from build123d import *

# Parameters (mm, degrees)
EXTRUDE_1_DEPTH      = 18
EXTRUDE_2_DEPTH      = 11
SKETCH_3_R           = 1
SKETCH_3_R_2         = 1.5
CUT_EXTRUDE_1_DEPTH  = 31
SKETCH_4_R           = 3
CUT_EXTRUDE_2_DEPTH  = 7
CUT_EXTRUDE_START    = -7
SKETCH_5_R           = 3
CUT_EXTRUDE_3_DEPTH  = 7
SKETCH_6_R           = 2.5
EXTRUDE_3_DEPTH      = 16
CUT_EXTRUDE_START_2  = -9
CUT_EXTRUDE_4_DEPTH  = 9
EXTRUDE_START        = 16
SKETCH_8_R           = 2.5
EXTRUDE_4_DEPTH      = 16
CUT_EXTRUDE_5_DEPTH  = 9
EXTRUDE_5_DEPTH      = 5
SKETCH_11_R          = 1
CUT_EXTRUDE_6_DEPTH  = 14
SKETCH_12_R          = 2
EXTRUDE_6_DEPTH      = 2
SKETCH_13_R          = 2
CUT_EXTRUDE_7_DEPTH  = 5
EXTRUDE_START_2      = 3
SKETCH_14_R          = 1.4
EXTRUDE_8_DEPTH      = 3
CUT_EXTRUDE_8_DEPTH  = 22
CUT_EXTRUDE_9_DEPTH  = 11
SKETCH_18_W          = 4.5245364
SKETCH_18_H          = 2
EXTRUDE_9_DEPTH      = 3
SKETCH_19_W          = 2
SKETCH_19_H          = 1
CUT_EXTRUDE_10_DEPTH = 8
SKETCH_20_W          = 2
SKETCH_20_H          = 1
CUT_EXTRUDE_11_DEPTH = 8
EXTRUDE_START_3      = 25
EXTRUDE_10_DEPTH     = 25
CUT_EXTRUDE_13_DEPTH = 1
EXTRUDE_11_DEPTH     = 3
EXTRUDE_11_DRAFT     = 20
SKETCH_25_R          = 5
EXTRUDE_12_DEPTH     = 2
CUT_EXTRUDE_START_3  = -2
CUT_EXTRUDE_14_DEPTH = 2
CUT_EXTRUDE_START_4  = -14
CUT_EXTRUDE_15_DEPTH = 14
CUT_EXTRUDE_16_DEPTH = 14
SKETCH_32_R          = 1
EXTRUDE_13_DEPTH     = 1


with BuildPart() as part:
    # 草图1 → 凸台-拉伸1 (new body)
    with BuildSketch(Plane.XY):
        with BuildLine():
            Line((0, 0), (-8, 0))
            ThreePointArc((-8, 0), (-10.121320344, 0.878679656), (-11, 3))
            Line((-11, 3), (-11, 32))
            Line((-11, 32), (11, 32))
            Line((11, 32), (11, 3))
            ThreePointArc((11, 3), (10.121320344, 0.878679656), (8, 0))
            Line((8, 0), (0, 0))
        make_face()
    extrude(amount=EXTRUDE_1_DEPTH)

    # 草图2 → 凸台-拉伸2 (add)
    with BuildSketch(Plane(origin=(0, 32, 0), x_dir=(1, 0, 0), z_dir=(0, 1, 0))):
        with BuildLine():
            Line((7.5, -18), (-7.5, -18))
            ThreePointArc((-7.5, -18), (-11.02081528, -9.5), (-7.5, -1))
            Line((-7.5, -1), (0, -1))
            Line((0, -1), (7.5, -1))
            ThreePointArc((7.5, -1), (11.02081528, -9.5), (7.5, -18))
        make_face()
    extrude(amount=EXTRUDE_2_DEPTH)

    # 草图3 → 切除-拉伸1 (cut)
    with BuildSketch(Plane.XY.offset(18)):
        with Locations((9, 30)):
            Circle(SKETCH_3_R)
        with Locations((8.5, 26.5)):
            Circle(SKETCH_3_R_2)
        with Locations((-8.5, 26.5)):
            Circle(SKETCH_3_R_2)
        with Locations((-9, 30)):
            Circle(SKETCH_3_R)
    extrude(amount=-CUT_EXTRUDE_1_DEPTH, mode=Mode.SUBTRACT)

    # 草图4 → 切除-拉伸2 (cut)
    with BuildSketch(Plane.XY.offset(18)):
        with Locations((0, 13)):
            Circle(SKETCH_4_R)
    extrude(amount=-CUT_EXTRUDE_2_DEPTH, mode=Mode.SUBTRACT)

    # 草图5 → 切除-拉伸3 (cut)
    with BuildSketch(Plane(origin=(0, 0, 0), x_dir=(-1, 0, 0), z_dir=(0, 0, -1)).offset(CUT_EXTRUDE_START)):
        with Locations(Location((0, 13, 0), (0, 0, 180))):
            Circle(SKETCH_5_R)
    extrude(amount=CUT_EXTRUDE_3_DEPTH, mode=Mode.SUBTRACT)

    # 草图6 → 凸台-拉伸3 (add)
    with BuildSketch(Plane.XY.offset(11)):
        with Locations((0, 13)):
            Circle(SKETCH_6_R)
    extrude(amount=EXTRUDE_3_DEPTH)

    # 草图7 → 切除-拉伸4 (cut)
    with BuildSketch(Plane.XY.offset(27).offset(CUT_EXTRUDE_START_2)):
        with BuildLine():
            Line((0, 15.5), (2.5, 13))
            ThreePointArc((2.5, 13), (1.767766953, 14.767766953), (0, 15.5))
        make_face()
        with BuildLine():
            Line((-2.5, 13), (0, 10.5))
            ThreePointArc((0, 10.5), (-1.767766953, 11.232233047), (-2.5, 13))
        make_face()
    extrude(amount=CUT_EXTRUDE_4_DEPTH, mode=Mode.SUBTRACT)

    # 草图8 → 凸台-拉伸4 (add)
    with BuildSketch(Plane(origin=(0, 0, 7), x_dir=(-1, 0, 0), z_dir=(0, 0, -1)).offset(EXTRUDE_START)):
        with Locations(Location((0, 13, 0), (0, 0, 180))):
            Circle(SKETCH_8_R)
    extrude(amount=-EXTRUDE_4_DEPTH)

    # 草图9 → 切除-拉伸5 (cut)
    with BuildSketch(Plane(origin=(0, 0, -9), x_dir=(-1, 0, 0), z_dir=(0, 0, -1))):
        with BuildLine():
            Line((0, 15.5), (2.5, 13))
            ThreePointArc((2.5, 13), (1.767766953, 14.767766953), (0, 15.5))
        make_face()
        with BuildLine():
            Line((-2.5, 13), (0, 10.5))
            ThreePointArc((0, 10.5), (-1.767766953, 11.232233047), (-2.5, 13))
        make_face()
    extrude(amount=-CUT_EXTRUDE_5_DEPTH, mode=Mode.SUBTRACT)

    # 草图10 → 凸台-拉伸5 (add)
    with BuildSketch(Plane.XZ):
        Polygon((-2.5, 9), (-2.5, 10.5), (2.5, 10.5), (2.5, 7.5), (-2.5, 7.5), align=None)
    extrude(amount=EXTRUDE_5_DEPTH)

    # 草图11 → 切除-拉伸6 (cut)
    with BuildSketch(Plane.XY.offset(10.5)):
        with Locations((0, -2.5)):
            Circle(SKETCH_11_R)
    extrude(amount=-CUT_EXTRUDE_6_DEPTH, mode=Mode.SUBTRACT)

    # 草图12 → 凸台-拉伸6 (add)
    with BuildSketch(Plane(origin=(0, 0, 0), x_dir=(-1, 0, 0), z_dir=(0, 0, -1))):
        with Locations(Location((0, 22, 0), (0, 0, 180))):
            Circle(SKETCH_12_R)
    extrude(amount=EXTRUDE_6_DEPTH)

    # 草图13 → 切除-拉伸7 (cut)
    with BuildSketch(Plane(origin=(0, 0, 0), x_dir=(-1, 0, 0), z_dir=(0, 0, -1))):
        with Locations((-6.646802627, 28.881218783)):
            Circle(SKETCH_13_R)
        with Locations((6.646802627, 28.881218783)):
            Circle(SKETCH_13_R)
    extrude(amount=-CUT_EXTRUDE_7_DEPTH, mode=Mode.SUBTRACT)

    # 草图14 → 凸台-拉伸8 (add)
    # profile 1 of 2: a face of its own
    with BuildSketch(Plane(origin=(0, 0, 5), x_dir=(-1, 0, 0), z_dir=(0, 0, -1)).offset(EXTRUDE_START_2)):
        with BuildLine():
            ThreePointArc((-8.638081379, 29.067790307), (-8.61386249, 28.519728121), (-8.441642649, 27.998864377))
            ThreePointArc((-8.441642649, 27.998864377), (-7.578736532, 27.683754038), (-7.061366244, 26.924656234))
            ThreePointArc((-7.061366244, 26.924656234), (-4.726868568, 29.441444815), (-8.048546627, 30.307792916))
            ThreePointArc((-8.048546627, 30.307792916), (-8.096873145, 29.570626173), (-8.638081379, 29.067790307))
        make_face()
        with Locations((-6.646802627, 28.881218783)):
            Circle(SKETCH_14_R, mode=Mode.SUBTRACT)
    # profile 2 of 2: a face of its own
    with BuildSketch(Plane(origin=(0, 0, 5), x_dir=(-1, 0, 0), z_dir=(0, 0, -1)).offset(EXTRUDE_START_2)):
        with BuildLine():
            ThreePointArc((7.061366244, 26.924656234), (4.726868568, 29.441444815), (8.048546627, 30.307792916))
            ThreePointArc((8.048546627, 30.307792916), (8.096873145, 29.570626173), (8.638081379, 29.067790307))
            ThreePointArc((8.638081379, 29.067790307), (8.61386249, 28.519728121), (8.441642649, 27.998864377))
            ThreePointArc((8.441642649, 27.998864377), (7.578736532, 27.683754038), (7.061366244, 26.924656234))
        make_face()
        with Locations(Location((6.646802627, 28.881218783, 0), (0, 0, 180))):
            Circle(SKETCH_14_R, mode=Mode.SUBTRACT)
    extrude(amount=-EXTRUDE_8_DEPTH)

    # 草图16 → 切除-拉伸8 (cut)
    with BuildSketch(Plane(origin=(0, 0, 1), x_dir=(-1, 0, 0), z_dir=(0, 0, -1))):
        Polygon((0, 36), (3.5, 36), (3.5, 38), (-3.5, 38), (-3.5, 36), align=None)
    extrude(amount=-CUT_EXTRUDE_8_DEPTH, mode=Mode.SUBTRACT)

    # 草图17 → 切除-拉伸9 (cut)
    with BuildSketch(Plane(origin=(0, 43, 0), x_dir=(1, 0, 0), z_dir=(0, 1, 0))):
        with BuildLine():
            Line((7.5, -2), (-7.5, -2))
            ThreePointArc((-7.5, -2), (-10.606601718, -9.5), (-7.5, -17))
            Line((-7.5, -17), (7.5, -17))
            ThreePointArc((7.5, -17), (10.606601718, -9.5), (7.5, -2))
        make_face()
    extrude(amount=-CUT_EXTRUDE_9_DEPTH, mode=Mode.SUBTRACT)

    # 草图18 → 凸台-拉伸9 (add)
    with BuildSketch(Plane(origin=(0, 0, 1), x_dir=(-1, 0, 0), z_dir=(0, 0, -1))):
        with Locations((0, 39)):
            Rectangle(SKETCH_18_W, SKETCH_18_H)
    extrude_9 = extrude(amount=EXTRUDE_9_DEPTH)

    # 草图19 → 切除-拉伸10 (cut)
    with BuildSketch(Plane(origin=(2.2622682, 0, 0), x_dir=(0, 0, -1), z_dir=(1, 0, 0))):
        with Locations((0, 38.5)):
            Rectangle(SKETCH_19_W, SKETCH_19_H)
    extrude(amount=-CUT_EXTRUDE_10_DEPTH, mode=Mode.SUBTRACT)

    # 镜向2: 凸台-拉伸9 across plane
    add(extrude_9.mirror(Plane.XY.offset(9.5)))

    # 草图20 → 切除-拉伸11 (cut)
    with BuildSketch(Plane.ZY.offset(2.2622682)):
        with Locations((19, 38.5)):
            Rectangle(SKETCH_20_W, SKETCH_20_H)
    extrude(amount=-CUT_EXTRUDE_11_DEPTH, mode=Mode.SUBTRACT)

    # 草图21 → 凸台-拉伸10 (add)
    with BuildSketch(Plane(origin=(0, 32, 0), x_dir=(1, 0, 0), z_dir=(0, 1, 0)).offset(EXTRUDE_START_3)):
        with BuildLine():
            Line((7.5, -2), (-7.5, -2))
            ThreePointArc((-7.5, -2), (-10.606601718, -9.5), (-7.5, -17))
            Line((-7.5, -17), (7.5, -17))
            ThreePointArc((7.5, -17), (10.606601718, -9.5), (7.5, -2))
        make_face()
    extrude(amount=-EXTRUDE_10_DEPTH)

    # 草图23 → 切除-拉伸13 (cut)
    with BuildSketch(Plane(origin=(0, 57, 0), x_dir=(1, 0, 0), z_dir=(0, 1, 0))):
        with BuildLine():
            Line((-10.496934744, -7.978697601), (-7.496934744, -7.978697601))
            ThreePointArc((-7.496934744, -7.978697601), (-6.866790657, -9.5), (-7.496934744, -11.021302399))
            Line((-7.496934744, -11.021302399), (-10.496934744, -11.021302399))
            ThreePointArc((-10.496934744, -11.021302399), (-10.606601718, -9.5), (-10.496934744, -7.978697601))
        make_face()
        with BuildLine():
            Line((7.496934744, -11.021302399), (10.496934744, -11.021302399))
            ThreePointArc((10.496934744, -11.021302399), (10.606601718, -9.5), (10.496934744, -7.978697601))
            Line((10.496934744, -7.978697601), (7.496934744, -7.978697601))
            ThreePointArc((7.496934744, -7.978697601), (6.866790657, -9.5), (7.496934744, -11.021302399))
        make_face()
    extrude(amount=-CUT_EXTRUDE_13_DEPTH, mode=Mode.SUBTRACT)


with BuildPart() as extrude_11_tool:
    # 草图24 → 凸台-拉伸11 (with draft: the straight prism first)
    with BuildSketch(Plane(origin=(0, 57, 0), x_dir=(1, 0, 0), z_dir=(0, 1, 0))):
        with BuildLine():
            Line((7.5, -2), (-7.5, -2))
            ThreePointArc((-7.5, -2), (-10.289850602, -9.5), (-7.5, -17))
            Line((-7.5, -17), (7.5, -17))
            ThreePointArc((7.5, -17), (10.289850602, -9.5), (7.5, -2))
        make_face()
    extrude(amount=EXTRUDE_11_DEPTH)
    # 凸台-拉伸11: the draft: its side faces are tilted about the plane it starts from
    extrude_11_sides = [extrude_11_tool.faces().sort_by_distance(p)[0] for p in [
        (0, 58.5, 2),
        (-10.289850602, 58.5, 9.5),
        (0, 58.5, 17),
        (10.289850602, 58.5, 9.5),
    ]]
    draft(extrude_11_sides, Plane(origin=(0, 57, 0), x_dir=(1, 0, 0), z_dir=(0, 1, 0)), EXTRUDE_11_DRAFT)


with BuildPart() as part_1:
    add(part.part)

    # 凸台-拉伸11: add extrude_11_tool
    add(extrude_11_tool.part)

    # 草图25 → 凸台-拉伸12 (add)
    with BuildSketch(Plane(origin=(0, 60, 0), x_dir=(1, 0, 0), z_dir=(0, 1, 0))):
        with Locations(Location((0, -9.5, 0), (0, 0, 90))):
            Circle(SKETCH_25_R)
    extrude(amount=EXTRUDE_12_DEPTH)

    # 草图26 → 切除-拉伸14 (cut)
    with BuildSketch(Plane(origin=(0, 62, 0), x_dir=(1, 0, 0), z_dir=(0, 1, 0)).offset(CUT_EXTRUDE_START_3)):
        with BuildLine():
            Line((3.977952818, -6.470826618), (-3.977952818, -6.470826618))
            ThreePointArc((-3.977952818, -6.470826618), (0, -4.5), (3.977952818, -6.470826618))
        make_face()
    extrude(amount=CUT_EXTRUDE_14_DEPTH, mode=Mode.SUBTRACT)

    # 草图30 → 切除-拉伸15 (cut)
    with BuildSketch(Plane.XZ.offset(-57).offset(CUT_EXTRUDE_START_4)):
        with BuildLine():
            Line((7.496934744, 7.978697601), (10.496934744, 7.978697601))
            Line((10.496934744, 7.978697601), (10.496934744, 11.021302399))
            Line((10.496934744, 11.021302399), (7.496934744, 11.021302399))
            ThreePointArc((7.496934744, 11.021302399), (6.866790657, 9.5), (7.496934744, 7.978697601))
        make_face()
        with BuildLine():
            Line((-10.496934744, 11.021302399), (-7.496934744, 11.021302399))
            ThreePointArc((-7.496934744, 11.021302399), (-6.866790657, 9.5), (-7.496934744, 7.978697601))
            Line((-7.496934744, 7.978697601), (-10.496934744, 7.978697601))
            Line((-10.496934744, 7.978697601), (-10.496934744, 11.021302399))
        make_face()
    extrude(amount=CUT_EXTRUDE_15_DEPTH, mode=Mode.SUBTRACT)

    # 草图31 → 切除-拉伸16 (cut)
    with BuildSketch(Plane(origin=(0, 62, 0), x_dir=(1, 0, 0), z_dir=(0, 1, 0))):
        with BuildLine():
            Line((2, -12.67407861), (-2, -12.67407861))
            ThreePointArc((-2, -12.67407861), (-2.354738624, -12.319339986), (-2, -11.964601361))
            Line((-2, -11.964601361), (2, -11.964601361))
            ThreePointArc((2, -11.964601361), (2.354738624, -12.319339986), (2, -12.67407861))
        make_face()
    extrude(amount=-CUT_EXTRUDE_16_DEPTH, mode=Mode.SUBTRACT)

    # 草图32 → 凸台-拉伸13 (add)
    with BuildSketch(Plane(origin=(0, 62, 0), x_dir=(1, 0, 0), z_dir=(0, 1, 0))):
        with Locations(Location((0, -9.5, 0), (0, 0, 90))):
            Circle(SKETCH_32_R)
    extrude(amount=EXTRUDE_13_DEPTH)


solid = part_1.part
Read the model definition and answer for the solid it produces. Units are mm, in the model's axes. A direction names the side the tool comes from. Round coordinates to 2 decimals unless told otherwise and drop trailing zeros. Write each loop counter-clockwise with the first axis right and the second up, starting at its lowest first coordinate (ties: lowest second). Pieces come first, ordered by that corner, then holes.
Q1. Find section A-A on y = 50.5. Determine the outline of the cut face in (x, z), and give its area (3 significant figures).
Values:
outline: (-7.5, 2) - (7.5, 2) arc R10.61 ccw to (7.5, 17) - (-7.5, 17) arc R10.61 ccw to start; hole (-2, 11.96) - (2, 11.96) arc R0.35 ccw to (2, 12.67) - (-2, 12.67) arc R0.35 ccw to start
area: 286 mm2
Q2. Straight lines are drawn through the part: line 1 (X direction, y = 30, z = 7.25); line 2 (X direction, y = 26.5, z = 13.75); line 3 (Y direction, x = 0, z = 1.5). For each, find the intervals that lie inside material, in ascending order.
Values:
line 1: x = -11 to -10, -8 to 8, 10 to 11
line 2: x = -11 to -10, -7 to 7, 10 to 11
line 3: y = 0 to 10, 10.5 to 15.5, 16 to 36, 38 to 43
Q3. Find section D-D on y = 2. Determine the outline of the cut face in (x, z), and give its area (3 significant figures).
Values:
outline: (-10.83, 0) - (10.83, 0) - (10.83, 18) - (-10.83, 18) - close
area: 390 mm2
Q4. Find section B-B on z = 22. Determine the outline of the cut face in (x, y), and give its area (3 significant figures).
Values:
outline: (-2.5, 13) - (0, 10.5) arc R2.5 ccw to (2.5, 13) - (0, 15.5) arc R2.5 ccw to start
area: 16.1 mm2
Q5. The mould has two halves that part along X. Classify faces 6 (the face through (-0.1, 38.6, 1)), 7 (the face through (-2.262, 39.2, 19.8)), 8 (the face through (0, 55, 12.674)): released by +X, released by -X, zero draft, split by the parting line, or undercut.
Values:
face 6: zero draft
face 7: released by -X
face 8: undercut
Q6. Flat-ended cylindrical pins translate along their axes: P1, Ø6, axis at x = -4.5, y = 38.5, coming from the -Z side; P2, Ø12, axis at x = 7, y = 33, coming from the -Z side; P3, Ø4, axis at y = 41, z = 2.5, coming from the -X side. Find the tip coordinate at first contact, or state that the pin passes through.
Values:
P1: stops at z = -2
P2: stops at z = 0
P3: stops at x = -9.93
Q7. Find section C-C on y = 11.5. Determine the outline of the cut face in (x, z), and give its area (3 significant figures).
Values:
outline: (-11, 0) - (-2.6, 0) - (-2.6, 7) - (-2, 7) - (-2, -9) - (1, -9) - (1, 0) - (2, 0) - (2, 7) - (2.6, 7) - (2.6, 0) - (11, 0) - (11, 18) - (2.6, 18) - (2.6, 11) - (2, 11) - (2, 27) - (-1, 27) - (-1, 18) - (-2, 18) - (-2, 11) - (-2.6, 11) - (-2.6, 18) - (-11, 18) - close
area: 433 mm2
Q8. A tool of negligible diameter and unlimited length cuts with its end or side. For faces 1 (the face through (0, 39, 0)), 2 (the face through (-0.65, 10.07, 14.55)), 3 (the face through (5, 29, 2)), 4 (the face through (9, 58, 7.979)), 5 (the face through (-9, 56, 9)), from which of +Z, -Z, +X, -X, +Y, -Y can it reach the whole face along a straight path? Write none if from no direction.
Values:
face 1: +X, -X
face 2: +Z
face 3: -Z
face 4: +X, +Y
face 5: -X, +Y
